For this review, take the finished solid that the model builds, in its own axes (mm). Give positions to 0.01 mm unless a question says otherwise; leave off trailing zeros. Loops run counter-clockwise (first coordinate to the right, second up) from the corner with the lowest first, then second, coordinate; pieces in that order, holes last. Notation, with made-up numbers: (11, 76.5) - (17, 76.5) arc R31 cw to (17, 113.5) - close; hole circle Ø1 at (-10.5, 17). An arc over 180 degrees is marked (long way). Use CSV: the item, a comma, the result in double quotes. Start each with the question number.
1. Take a section at D-D on z = -60.5. Give the boundary of the cut face in (x, y).
2. Take a section at C-C on x = 46.5. Give the boundary of the cut face in (y, z), plus the area to 3 significant figures.
3. Take a section at B-B on y = 5.25. Give the boundary of the cut face in (x, z), plus the area to 3 significant figures.
4. Wall thickness on line 1 (X direction, y = 1.25, z = -37.5); line 2 (Z direction, x = 13.5, y = 6.25); line 3 (Z direction, x = 19.5, y = 5.5): over which ranges is each line inside the solid? List them lowest first.
5. Take a section at A-A on z = -38.1. Give the boundary of the cut face in (x, y).
6. For pin 1 (2 mm diameter, centred on x = 9, z = -36.5, fed in from -Y); pin 2 (2 mm diameter, centred on x = 29.337, z = -38.1, fed in from +Y); pin 3 (1 mm diameter, centred on y = 1, z = -63, fed in from -X), all flat-tipped, find the tip position at first contact; note any pin that passes through.
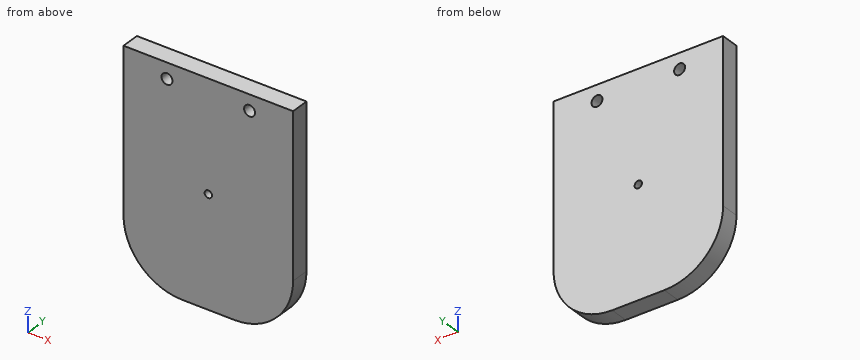
```python
from build123d import *

# Parameters (mm, degrees)
SKETCH1_W           = 58.674
SKETCH1_H           = 76.2
BOSS_EXTRUDE1_DEPTH = 6.35
CUT_EXTRUDE1_DEPTH  = 97.381537527
SKETCH3_W           = 58.674
SKETCH3_H           = 6.35
BOSS_EXTRUDE2_DEPTH = 7.62
SKETCH4_W           = 15.24
SKETCH4_H           = 7.62
CUT_EXTRUDE2_DEPTH  = 97.381537527
FILLET1_R           = 3.175
SKETCH5_R           = 2.54
CUT_EXTRUDE3_DEPTH  = 88.939040568
FILLET2_R           = 20.32
SKETCH7_W           = 58.92775625
SKETCH7_H           = 8.241690561
CUT_EXTRUDE4_DEPTH  = 97.381537527
SKETCH8_R           = 1.89865
CUT_EXTRUDE5_DEPTH  = 97.381537527


with BuildPart() as part:
    # Sketch1 → Boss-Extrude1 (new body)
    with BuildSketch(Plane(origin=(0, 0, 0), x_dir=(1, 0, 0), z_dir=(0, 1, 0))):
        with Locations((29.337, 38.1)):
            Rectangle(SKETCH1_W, SKETCH1_H)
    extrude(amount=BOSS_EXTRUDE1_DEPTH)

    # Sketch2 → Cut-Extrude1 (cut, through all)
    with BuildSketch(Plane(origin=(0, 6.35, 0), x_dir=(1, 0, 0), z_dir=(0, 1, 0))):
        with BuildLine():
            ThreePointArc((30.607, 38.1), (29.337, 39.37), (28.067, 38.1))
            Line((28.067, 38.1), (30.607, 38.1))
        make_face()
        with BuildLine():
            Line((30.607, 38.1), (28.067, 38.1))
            ThreePointArc((28.067, 38.1), (29.337, 36.83), (30.607, 38.1))
        make_face()
    extrude(amount=-CUT_EXTRUDE1_DEPTH, mode=Mode.SUBTRACT)

    # Sketch3 → Boss-Extrude2 (add)
    with BuildSketch(Plane.XY):
        with Locations((29.337, 3.175)):
            Rectangle(SKETCH3_W, SKETCH3_H)
    extrude(amount=BOSS_EXTRUDE2_DEPTH)

    # Sketch4 → Cut-Extrude2 (cut, through all)
    with BuildSketch(Plane(origin=(0, 6.35, 0), x_dir=(1, 0, 0), z_dir=(0, 1, 0))):
        with Locations((7.62, -3.81)):
            Rectangle(SKETCH4_W, SKETCH4_H)
        with Locations((29.337, -3.81)):
            Rectangle(SKETCH4_W, SKETCH4_H)
        with Locations((51.054, -3.81)):
            Rectangle(SKETCH4_W, SKETCH4_H)
    extrude(amount=-CUT_EXTRUDE2_DEPTH, mode=Mode.SUBTRACT)

    # Fillet1
    fillet1_edges = [part.edges().sort_by_distance(p)[0] for p in [
        (40.1955, 0, 7.62),
        (40.1955, 6.35, 7.62),
        (18.4785, 0, 7.62),
        (18.4785, 6.35, 7.62),
    ]]
    fillet(fillet1_edges, radius=FILLET1_R - 0.0001)  # a hair under: the kernel refuses the full size

    # Sketch5 → Cut-Extrude3 (cut, through all)
    with BuildSketch(Plane(origin=(43.434, 0, 0), x_dir=(0, 0, -1), z_dir=(1, 0, 0))):
        with Locations((-4.445, 3.175)):
            Circle(SKETCH5_R)
    extrude(amount=-CUT_EXTRUDE3_DEPTH, mode=Mode.SUBTRACT)

    # Fillet2
    fillet2_edges = [part.edges().sort_by_distance(p)[0] for p in [
        (0, 3.175, -76.2),
        (58.674, 3.175, -76.2),
    ]]
    fillet(fillet2_edges, radius=FILLET2_R)

    # Sketch7 → Cut-Extrude4 (cut, through all)
    with BuildSketch(Plane(origin=(0, 6.35, 0), x_dir=(1, 0, 0), z_dir=(0, 1, 0))):
        with Locations((29.463878125, -4.120845281)):
            Rectangle(SKETCH7_W, SKETCH7_H)
    extrude(amount=-CUT_EXTRUDE4_DEPTH, mode=Mode.SUBTRACT)

    # Sketch8 → Cut-Extrude5 (cut, through all)
    with BuildSketch(Plane(origin=(0, 6.35, 0), x_dir=(1, 0, 0), z_dir=(0, 1, 0))):
        with Locations(Location((43.6245, 5.3975, 0), (0, 0, 270))):
            Circle(SKETCH8_R)
        with Locations(Location((15.0495, 5.3975, 0), (0, 0, 270))):
            Circle(SKETCH8_R)
    extrude(amount=-CUT_EXTRUDE5_DEPTH, mode=Mode.SUBTRACT)


solid = part.part
```
Check result:
1,outline,"(0.53, 0) - (58.14, 0) - (58.14, 6.35) - (0.53, 6.35) - close"
2,outline,"(0, -74.5) - (6.35, -74.5) - (6.35, 0) - (0, 0) - close"
2,area,"473 mm²"
3,outline,"(0, -55.88) arc R20.32 ccw to (20.32, -76.2) - (38.35, -76.2) arc R20.32 ccw to (58.67, -55.88) - (58.67, 0) - (0, 0) - close; hole circle Ø3.8 at (15.05, -5.4); hole circle Ø2.54 at (29.34, -38.1); hole circle Ø3.8 at (43.62, -5.4)"
3,area,"4,270 mm²"
4,line 1,"x = 0 to 28.22, 30.46 to 58.67"
4,line 2,"z = -75.02 to -6.49, -4.3 to 0"
4,line 3,"z = -76.18 to 0"
5,outline,"(0, 0) - (28.07, 0) - (28.07, 6.35) - (0, 6.35) - close; (30.61, 0) - (58.67, 0) - (58.67, 6.35) - (30.61, 6.35) - close"
6,pin 1,"stops at y = 0"
6,pin 2,"passes through"
6,pin 3,"stops at x = 1.11"
